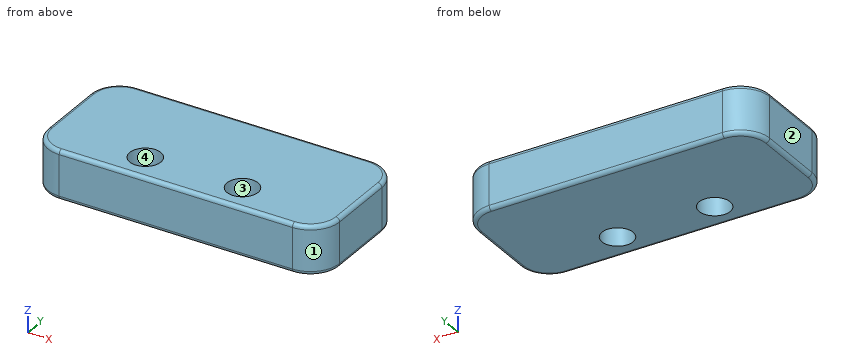
```python
from build123d import *

# Parameters (mm, degrees)
SKETCH1_W           = 30
SKETCH1_H           = 13
BOSS_EXTRUDE1_DEPTH = 5
SKETCH2_R           = 1.6
CUT_EXTRUDE1_DEPTH  = 34.075670817
FILLET1_R           = 3
FILLET2_R           = 0.4


with BuildPart() as part:
    # Sketch1 → Boss-Extrude1 (new body)
    with BuildSketch(Plane.XY):
        with Locations((15, -6.5)):
            Rectangle(SKETCH1_W, SKETCH1_H)
    extrude(amount=BOSS_EXTRUDE1_DEPTH)

    # Sketch2 → Cut-Extrude1 (cut, through all)
    with BuildSketch(Plane(origin=(0, 0, 0), x_dir=(-1, 0, 0), z_dir=(0, 0, -1))):
        with Locations((-20, -10)):
            Circle(SKETCH2_R)
        with Locations((-10, -10)):
            Circle(SKETCH2_R)
    extrude(amount=-CUT_EXTRUDE1_DEPTH, mode=Mode.SUBTRACT)

    # Fillet1
    fillet1_edges = [part.edges().sort_by_distance(p)[0] for p in [
        (0, 0, 2.5),
        (30, 0, 2.5),
        (30, -13, 2.5),
        (0, -13, 2.5),
    ]]
    fillet(fillet1_edges, radius=FILLET1_R)

    # Fillet2
    fillet2_edges = [part.edges().sort_by_distance(p)[0] for p in [
        (0, -6.5, 0),
        (0, -6.5, 5),
        (15, 0, 0),
        (30, -6.5, 0),
        (15, -13, 0),
        (29.121320344, -0.878679656, 0),
        (29.121320344, -12.121320344, 0),
        (0.878679656, -12.121320344, 0),
        (0.878679656, -0.878679656, 0),
        (15, 0, 5),
        (15, -13, 5),
        (30, -6.5, 5),
        (29.121320344, -0.878679656, 5),
        (29.121320344, -12.121320344, 5),
        (0.878679656, -12.121320344, 5),
        (0.878679656, -0.878679656, 5),
    ]]
    fillet(fillet2_edges, radius=FILLET2_R)


solid = part.part
```
Model file for the job. Use its own axes, mm. Face numbers are marked on the shaded views. Give positions to 0.01 mm unless a question says otherwise; leave off trailing zeros. Order: outer loops, then holes, each group sorted by start corner. A loop starts at its lowest first (then second) coordinate and runs counter-clockwise, first axis right, second up.
1) Saw through at C-C, the plane x = 20.5. Write the cut outline in (y, z).
2) Pin check, flat tip, straight feed: pin 1 (1 mm diameter, centred on y = -1.5, z = 3.5, fed in from +X). Stop position of the tip, or through.
3) Wall check: probe 1 along Y at (x, z) = (10, 0.75); probe 2 along X at (y, z) = (-9, 0.7); probe 3 along X at (y, z) = (-12, 2.3). Give the ranges that are in metal, low to high.
4) Mould opens along Y. For the marked faces 1, 2, 3 and 4 say: +Y half, -Y half, draft (parallel to the pull), parting line (faces both ways), or undercut.
5) Saw through at B-B, the plane z = 1.15. Write the cut outline in (x, y), then the cut area to 3 significant figures.
6) Saw through at A-A, the plane x = 10. Write the cut outline in (y, z), then the cut area to 3 significant figures.
Computed:
1. outline: (-13, 0.4) arc R0.4 ccw to (-12.6, 0) - (-11.52, 0) - (-11.52, 5) - (-12.6, 5) arc R0.4 ccw to (-13, 4.6) - close; (-8.48, 0) - (-0.4, 0) arc R0.4 ccw to (0, 0.4) - (0, 4.6) arc R0.4 ccw to (-0.4, 5) - (-8.48, 5) - close
2. pin 1: stops at x = 29.83
3. probe 1: y = -13 to -11.6, -8.4 to 0
3. probe 2: x = 0 to 8.75, 11.25 to 18.75, 21.25 to 30
3. probe 3: x = 0.76 to 29.24
4. face 1: -Y half
4. face 2: draft
4. face 3: undercut
4. face 4: undercut
5. outline: (0, -10) arc R3 ccw to (3, -13) - (27, -13) arc R3 ccw to (30, -10) - (30, -3) arc R3 ccw to (27, 0) - (3, 0) arc R3 ccw to (0, -3) - close; hole circle Ø3.2 at (10, -10); hole circle Ø3.2 at (20, -10)
5. area: 366 mm2
6. outline: (-13, 0.4) arc R0.4 ccw to (-12.6, 0) - (-11.6, 0) - (-11.6, 5) - (-12.6, 5) arc R0.4 ccw to (-13, 4.6) - close; (-8.4, 0) - (-0.4, 0) arc R0.4 ccw to (0, 0.4) - (0, 4.6) arc R0.4 ccw to (-0.4, 5) - (-8.4, 5) - close
6. area: 48.9 mm2
